from build123d import *

# Parameters (mm, degrees)
SKETCH2_R                                       = 37.5
BOSS_EXTRUDE1_DEPTH                             = 13.97
CSK_FOR_M6_FLAT_HEAD_MACHINE_SCREW1_D           = 6.6
CSK_FOR_M6_FLAT_HEAD_MACHINE_SCREW1_CSINK_D     = 12.6
CSK_FOR_M6_FLAT_HEAD_MACHINE_SCREW1_CSINK_ANGLE = 90
M5X0_8_TAPPED_HOLE1_D                           = 4.2
M5X0_8_TAPPED_HOLE1_DEPTH                       = 12.192
M5X0_8_TAPPED_HOLE1_TIP                         = 1.2618073
SKETCH1_R                                       = 1.9685
CUT_EXTRUDE1_DEPTH                              = 5.08
SKETCH1_3_W                                     = 12.7
SKETCH1_3_H                                     = 6.35
POGO_PINS_DEPTH                                 = 3.048
SKETCH8_R                                       = 3
CUT_EXTRUDE2_DEPTH                              = 10.16
SKETCH9_R                                       = 37.5
SKETCH9_R_2                                     = 34.96
LIP_DEPTH                                       = 2.54
CHAMFER1_SIZE                                   = 0.508


with BuildPart() as part:
    # Sketch2 → Boss-Extrude1 (new body)
    with BuildSketch(Plane(origin=(0, 0, 0), x_dir=(1, 0, 0), z_dir=(0, 1, 0))):
        Circle(SKETCH2_R)
    extrude(amount=BOSS_EXTRUDE1_DEPTH)

    # CSK for M6 Flat Head Machine Screw1 (through all)
    with Locations(Plane(origin=(0, 0, 0), x_dir=(-1, 0, 0), z_dir=(0, -1, 0))):
        with Locations((-17.67766953, 17.67766953), (17.67766953, 17.67766953), (17.67766953, -17.67766953), (-17.67766953, -17.67766953)):
            CounterSinkHole(CSK_FOR_M6_FLAT_HEAD_MACHINE_SCREW1_D / 2, CSK_FOR_M6_FLAT_HEAD_MACHINE_SCREW1_CSINK_D / 2, counter_sink_angle=CSK_FOR_M6_FLAT_HEAD_MACHINE_SCREW1_CSINK_ANGLE)

    # M5x0.8 Tapped Hole1
    with Locations(Plane(origin=(0, 0, 0), x_dir=(-1, 0, 0), z_dir=(0, -1, 0))):
        with Locations((-27.305, 16.1925), (-27.305, -16.1925), (27.305, -16.1925), (27.305, 16.1925)):
            Hole(M5X0_8_TAPPED_HOLE1_D / 2, depth=M5X0_8_TAPPED_HOLE1_DEPTH)
            with Locations((0, 0, -(M5X0_8_TAPPED_HOLE1_DEPTH + M5X0_8_TAPPED_HOLE1_TIP / 2))):  # 118° drill point
                Cone(0, M5X0_8_TAPPED_HOLE1_D / 2, M5X0_8_TAPPED_HOLE1_TIP, mode=Mode.SUBTRACT)

    # Sketch1 → Cut-Extrude1 (cut)
    with BuildSketch(Plane(origin=(0, 0, 0), x_dir=(1, 0, 0), z_dir=(0, 1, 0))):
        with Locations((-30.515, 0)):
            Circle(SKETCH1_R)
    extrude(amount=CUT_EXTRUDE1_DEPTH, mode=Mode.SUBTRACT)

    # Sketch1_3 → Pogo pins (add)
    with BuildSketch(Plane(origin=(0, 0, 0), x_dir=(1, 0, 0), z_dir=(0, 1, 0))):
        with Locations((-12.5572, 0)):
            Rectangle(SKETCH1_3_W, SKETCH1_3_H)
    extrude(amount=-POGO_PINS_DEPTH)

    # Sketch8 → Cut-Extrude2 (cut)
    with BuildSketch(Plane(origin=(0, 13.97, 0), x_dir=(1, 0, 0), z_dir=(0, 1, 0))):
        with Locations((0, -25)):
            Circle(SKETCH8_R)
        with BuildLine():
            ThreePointArc((-15.875, -33.974025004), (0, -37.5), (15.875, -33.974025004))
            Line((15.875, -33.974025004), (-15.875, -33.974025004))
        make_face()
    extrude(amount=-CUT_EXTRUDE2_DEPTH, mode=Mode.SUBTRACT)

    # Sketch9 → Lip (add)
    with BuildSketch(Plane.XZ):
        Circle(SKETCH9_R)
        Circle(SKETCH9_R_2, mode=Mode.SUBTRACT)
    extrude(amount=LIP_DEPTH)

    # Chamfer1
    chamfer1_edges = [part.edges().sort_by_distance(p)[0] for p in [
        (-34.96, -2.54, 0),
    ]]
    chamfer(chamfer1_edges, length=CHAMFER1_SIZE)


solid = part.part
For this review, take the finished solid that the model builds, in its own axes (mm). A direction names the side the tool comes from. Round coordinates to 2 decimals unless told otherwise and drop trailing zeros. Write each loop counter-clockwise with the first axis right and the second up, starting at its lowest first coordinate (ties: lowest second). Pieces come first, ordered by that corner, then holes. Notation, with made-up numbers: (-40, 44.25) - (-29, 44.25) arc R13 ccw to (-29, 49.25) - close; hole circle Ø7 at (19, 49.25). An arc over 180 degrees is marked (long way). Use a Markdown table: item, result.
Q1. We need section C-C (x = 0). Give the boundary of the cut face in (y, z).
Derived:
| item | result |
|---|---|
| outline | (-2.54, -37.5) - (13.97, -37.5) - (13.97, 22) - (3.81, 22) - (3.81, 28) - (13.97, 28) - (13.97, 33.97) - (3.81, 33.97) - (3.81, 37.5) - (-2.54, 37.5) - (-2.54, 35.47) - (-2.03, 34.96) - (0, 34.96) - (0, -34.96) - (-2.03, -34.96) - (-2.54, -35.47) - close |
Q2. The part is to be moulded in two halves that separate along Z. For faces 1 (the flat face through (0, 9, 33.974)), 2 (the flat face through (0, 0, 0)), 3 (the flat face through (-1, 13.97, -2)), say which applies: pulls with the +Z half, pulls with the -Z half, needs draft (parallel to the pull), parting line crosses it, or undercut.
Derived:
| item | result |
|---|---|
| face 1 | pulls with the +Z half |
| face 2 | undercut |
| face 3 | needs draft |
Q3. Machinability: for faces 4 (the cylindrical face through (-20.974, 8.562, 17.533)), 5 (the flat face through (-6.207, -2, 0)), which of the approach directions +Z, -Z, +X, -X, +Y, -Y give a long, thin tool a straight path to every point of the face, cutting with its end or side? Answer none if there is none.
Derived:
| item | result |
|---|---|
| face 4 | +Y, -Y |
| face 5 | -Y |
Q4. We need section A-A (y = 1.75). State how many separate pieces and enclosed holes the cut face has, plus the area to 3 significant figures.
Derived:
| item | result |
|---|---|
| separate pieces | 1 |
| enclosed holes | 9 |
| area | 4,090 mm2 |
Q5. Clearance check with flat-ended pins moving along their axes: pin 1 (3 mm diameter, centred on x = -3.5, y = 4, fed in from +Z); pin 2 (2.5 mm diameter, centred on x = -11.5, y = -1, fed in from +Z); pin 3 (5.5 mm diameter, centred on x = 0, z = 25, fed in from +Y). State where each tip first meets the part, or that it passes through.
Derived:
| item | result |
|---|---|
| pin 1 | stops at z = 37.45 |
| pin 2 | stops at z = 36.07 |
| pin 3 | stops at y = 3.81 |
Q6. Wall thickness on line 1 along Z through (x, y) = (0, 10.25); line 2 along Z through (x, y) = (26.5, 4.5); line 3 along Y through (x, z) = (9, 13.5): over which ranges is each line inside the solid? List them lowest first.
Derived:
| item | result |
|---|---|
| line 1 | z = -37.5 to 22, 28 to 33.97 |
| line 2 | z = -26.53 to -18.13, -14.25 to 14.25, 18.13 to 26.53 |
| line 3 | y = 0 to 13.97 |
Q7. We need section B-B (z = 0). Give the boundary of the cut face in (x, y).
Derived:
| item | result |
|---|---|
| outline | (-37.5, -2.54) - (-35.47, -2.54) - (-34.96, -2.03) - (-34.96, 0) - (-32.48, 0) - (-32.48, 5.08) - (-28.55, 5.08) - (-28.55, 0) - (-18.91, 0) - (-18.91, -3.05) - (-6.21, -3.05) - (-6.21, 0) - (34.96, 0) - (34.96, -2.03) - (35.47, -2.54) - (37.5, -2.54) - (37.5, 13.97) - (-37.5, 13.97) - close |
